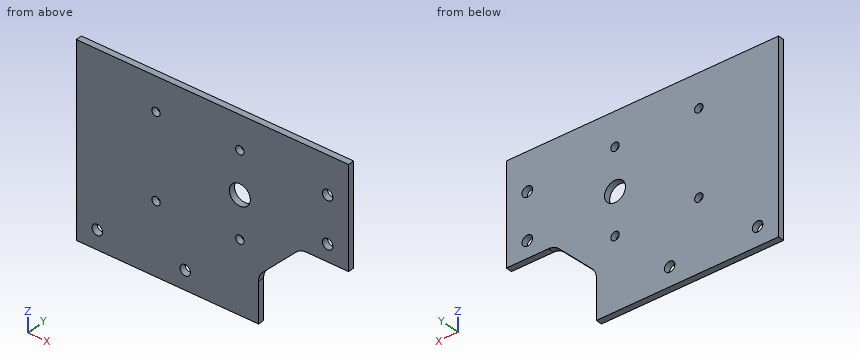
from build123d import *

# Parameters (mm, degrees)
SKETCH1_R           = 2.5
BOSS_EXTRUDE1_DEPTH = 3
SKETCH2_R           = 2
SKETCH2_R_2         = 5
CUT_EXTRUDE2_DEPTH  = 3


with BuildPart() as part:
    # Sketch1 → Boss-Extrude1 (new body)
    with BuildSketch(Plane(origin=(0, 0, 0), x_dir=(1, 0, 0), z_dir=(0, 1, 0))):
        with BuildLine():
            Line((0, -42), (-20.100505063, -42))
            ThreePointArc((-20.100505063, -42), (-22.77928909, -41.467156728), (-25.050252532, -39.949747468))
            Line((-25.050252532, -39.949747468), (-40.949747468, -24.050252532))
            ThreePointArc((-40.949747468, -24.050252532), (-42.467156728, -21.77928909), (-43, -19.100505063))
            Line((-43, -19.100505063), (-43, 0))
            Line((-43, 0), (-130, 0))
            Line((-130, 0), (-130, -90))
            Line((-130, -90), (0, -90))
            Line((0, -90), (0, -42))
        make_face()
        with Locations(Location((-78, -9, 0), (0, 0, 270))):
            Circle(SKETCH1_R, mode=Mode.SUBTRACT)
        with Locations(Location((-120, -9, 0), (0, 0, 270))):
            Circle(SKETCH1_R, mode=Mode.SUBTRACT)
        with Locations(Location((-10, -50, 0), (0, 0, 270))):
            Circle(SKETCH1_R, mode=Mode.SUBTRACT)
        with Locations(Location((-10, -72, 0), (0, 0, 270))):
            Circle(SKETCH1_R, mode=Mode.SUBTRACT)
    extrude(amount=BOSS_EXTRUDE1_DEPTH)

    # Sketch2 → Cut-Extrude2 (cut)
    with BuildSketch(Plane(origin=(0, 0, 0), x_dir=(1, 0, 0), z_dir=(0, 1, 0))):
        with Locations(Location((-51.919512874, -74, 0), (0, 0, 270))):
            Circle(SKETCH2_R)
        with Locations(Location((-51.919512874, -54, 0), (0, 0, 270))):
            Circle(SKETCH2_R_2)
        with Locations(Location((-51.919512874, -34, 0), (0, 0, 270))):
            Circle(SKETCH2_R)
        with Locations(Location((-91.919512874, -34, 0), (0, 0, 270))):
            Circle(SKETCH2_R)
        with Locations(Location((-91.919512874, -74, 0), (0, 0, 270))):
            Circle(SKETCH2_R)
    extrude(amount=CUT_EXTRUDE2_DEPTH, mode=Mode.SUBTRACT)


solid = part.part
The model under review builds one solid part; all positions refer to its coordinate system, in mm. Round coordinates to 2 decimals unless told otherwise and drop trailing zeros. Loops run counter-clockwise (first coordinate to the right, second up) from the corner with the lowest first, then second, coordinate; pieces in that order, holes last. Notation, with made-up numbers: (79.25, -34) -> (127.25, -34) arc R9 ccw to (127.25, -19) -> close; hole circle Ø10 at (12, -23.5). An arc over 180 degrees is marked (long way). Write item = value, one per line. Start each with the question number.
Item 1: Take a section at D-D on y = 1.55. Count the separate pieces of the cut face and the enclosed holes in it, plus the area to 3 significant figures.
Item 2: To check wall thickness, follow L1, parallel to X at y = 1.95, z = 9; L2, parallel to Z at x = -92.5, y = 1.4; L3, parallel to X at y = 2, z = 74. State the ranges of each line that lie inside material, in increasing order.
Item 3: Take a section at A-A on x = -120. Give the boundary of the cut face in (y, z).
Item 4: Take a section at B-B on z = 9. Give the boundary of the cut face in (x, y), plus the area to 3 significant figures.
Item 5: Insertion check: pin 1 (3 mm diameter, centred on x = -91.92, z = 74, fed in from +Y). The pin has a flat end and moves straight along its axis. Give the tip position at first contact, or say it passes through.
Item 6: Take a section at C-C on x = -10. Give the boundary of the cut face in (y, z).
Result:
q1.separate_pieces = 1
q1.enclosed_holes = 9
q1.area = 9,890 mm²
q2.L1 = -130 to -122.5, -117.5 to -80.5, -75.5 to -43
q2.L2 = 0 to 32.09, 35.91 to 72.09, 75.91 to 90
q2.L3 = -130 to -93.92, -89.92 to -53.92, -49.92 to -11.5, -8.5 to 0
q3.outline = (0, 0) -> (3, 0) -> (3, 6.5) -> (0, 6.5) -> close; (0, 11.5) -> (3, 11.5) -> (3, 90) -> (0, 90) -> close
q4.outline = (-130, 0) -> (-122.5, 0) -> (-122.5, 3) -> (-130, 3) -> close; (-117.5, 0) -> (-80.5, 0) -> (-80.5, 3) -> (-117.5, 3) -> close; (-75.5, 0) -> (-43, 0) -> (-43, 3) -> (-75.5, 3) -> close
q4.area = 231 mm²
q5.pin_1 = through
q6.outline = (0, 42) -> (3, 42) -> (3, 47.5) -> (0, 47.5) -> close; (0, 52.5) -> (3, 52.5) -> (3, 69.5) -> (0, 69.5) -> close; (0, 74.5) -> (3, 74.5) -> (3, 90) -> (0, 90) -> close
